Can you work these out from the model? Positions are in its coordinate system, mm. Face numbers are marked on the shaded views. A direction names the side the tool comes from. Give positions to 0.01 mm unless a question says otherwise; leave off trailing zeros. Write each loop counter-clockwise with the first axis right and the second up, starting at its lowest first coordinate (ties: lowest second). Pieces come first, ordered by that corner, then holes.
from build123d import *

# Parameters (mm, degrees)
CUT_EXTRUDE1_DEPTH = 8.92734
CHAMFER1_SIZE      = 0.127
CHAMFER2_SIZE      = 0.127
FILLET1_R          = 0.508
FILLET2_R          = 0.2032


with BuildPart() as part:
    # Sketch1 → Revolve1 (revolve)
    with BuildSketch(Plane.XZ):
        Polygon((15.5575, 7.92734), (0, 7.92734), (0, 0), (14.2875, 0), (14.2875, 5.89534), (13.97, 5.89534), (13.97, 6.40334), (15.5575, 6.40334), align=None)
    revolve(axis=Axis((0, 0, 7.92734), (0, 0, -1)))

    # Sketch2 → Cut-Extrude1 (cut, through all)
    with BuildSketch(Plane(origin=(0, 0, 0), x_dir=(-1, 0, 0), z_dir=(0, 0, -1))):
        Polygon((3.666174209, 6.35), (-3.666174209, 6.35), (-7.332348419, 0), (-3.666174209, -6.35), (3.666174209, -6.35), (7.332348419, 0), align=None)
    extrude(amount=-CUT_EXTRUDE1_DEPTH, mode=Mode.SUBTRACT)

    # Chamfer1
    chamfer1_edges = [part.edges().sort_by_distance(p)[0] for p in [
        (-15.5575, 0, 6.40334),
    ]]
    chamfer(chamfer1_edges, length=CHAMFER1_SIZE)

    # Chamfer2
    chamfer2_edges = [part.edges().sort_by_distance(p)[0] for p in [
        (-15.5575, 0, 7.92734),
    ]]
    chamfer(chamfer2_edges, length=CHAMFER2_SIZE)

    # Fillet1
    fillet1_edges = [part.edges().sort_by_distance(p)[0] for p in [
        (-14.2875, 0, 0),
    ]]
    fillet(fillet1_edges, radius=FILLET1_R)

    # Fillet2
    fillet2_edges = [part.edges().sort_by_distance(p)[0] for p in [
        (-3.666174209, 6.35, 3.96367),
        (-7.332348419, 0, 3.96367),
        (-3.666174209, -6.35, 3.96367),
        (3.666174209, -6.35, 3.96367),
        (7.332348419, 0, 3.96367),
        (3.666174209, 6.35, 3.96367),
    ]]
    fillet(fillet2_edges, radius=FILLET2_R)


solid = part.part
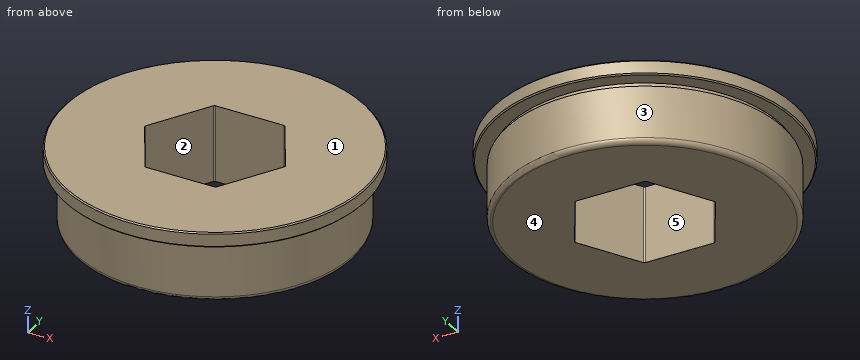
(1) For the marked faces 1 and 2, which set-ups out of +Z, -Z, +X, -X, +Y, -Y let a thin tool reach every point of the face, with its end or its side?
Returned:
face 1: +Z, +X, -X, +Y, -Y
face 2: +Z, -Z
(2) If I drill on L1, parallel to X at y = 2, z = 4; L2, parallel to Y at x = -3, z = 6.5; L3, parallel to Y at x = 1, z = 0.75, over which ranges is the centre line in solid material (lowest first)?
Returned:
L1: x = -14.15 to -6.18, 6.18 to 14.15
L2: y = -15.23 to -6.35, 6.35 to 15.23
L3: y = -14.25 to -6.35, 6.35 to 14.25
(3) Imagine slicing it at B-B, the plane x = 0. Write out the boundary of the cut face in (y, z), plus the area to 3 significant figures.
Returned:
outline: (-15.56, 6.53) - (-15.43, 6.4) - (-13.97, 6.4) - (-13.97, 5.9) - (-14.29, 5.9) - (-14.29, 0.51) arc R0.51 ccw to (-13.78, 0) - (-6.35, 0) - (-6.35, 7.93) - (-15.43, 7.93) - (-15.56, 7.8) - close; (6.35, 0) - (13.78, 0) arc R0.51 ccw to (14.29, 0.51) - (14.29, 5.9) - (13.97, 5.9) - (13.97, 6.4) - (15.43, 6.4) - (15.56, 6.53) - (15.56, 7.8) - (15.43, 7.93) - (6.35, 7.93) - close
area: 129 mm2
(4) Will these pins go through, and if not, where does the flat tip stop? P1, Ø1, axis at y = -4.5, z = 3.5, coming from the +X side; P2, Ø1, axis at x = 2.5, z = 3.5, coming from the -Y side; P3, Ø4, axis at x = 12.5, y = 5.5, coming from the -Z side; P4, Ø2, axis at y = 0.5, z = 4, coming from the +X side.
Returned:
P1: stops at x = 13.72
P2: stops at y = -14.15
P3: stops at z = 0
P4: stops at x = 14.29
(5) If we mould it in two halves opening along Y, with no side actions, what happens to the marked faces 3, 4 and 5? For each: +Y half, -Y half, draft (parallel to the pull), parting line (faces both ways), or undercut.
Returned:
face 3: parting line
face 4: draft
face 5: undercut
